Verification items for the finished model (mm, model axes). A direction names the side the tool comes from. Coordinates: 2 decimals unless noted, no trailing zeros. Order: outer loops, then holes, each group sorted by start corner. A loop starts at its lowest first (then second) coordinate and runs counter-clockwise, first axis right, second up. Notation, with made-up numbers: M -14,4 L -5,4 A18 ccw -5,21 Z; hole C 71.5,5 d11. An arc over 180 degrees is marked long. Return JSON: item names as keys, results as strings. Group by question number.
1. Section check D-D, the plane y = 3.9. Record the cut outline in (x, z), plus the area to 3 significant figures.
2. Section check A-A, the plane z = 2. Record the cut outline in (x, y), plus the area to 3 significant figures.
3. Section check C-C, the plane y = 2.1. Record the cut outline in (x, z).
4. Material ranges on line 1 along Y through (x, z) = (-1.25, 4.75); line 2 along X through (y, z) = (1.2, 9); line 3 along X through (y, z) = (1.7, 1), recorded low to high.
5. Set-up check for faces 4 (the flat face through (0, 3, 0)), 5 (the cylindrical face through (0, 2.8, 4.9)): record each of +Z, -Z, +X, -X, +Y, -Y from which the full face is reachable in a straight line by a thin tool's end or side.
6. Mould release check, pull along X, two halves, no side actions. Record for faces 1 (the flat face through (0.708, 2.008, 4.93)), 2 (the cylindrical face through (-4.715, 0.301, 5.07)), 3 (the cylindrical face through (4.699, 0.285, 5.07)): +X half, -X half, draft (parallel to the pull), parting line (faces both ways), or undercut.
7. Section check B-B, the plane x = 0. Record the cut outline in (y, z), plus the area to 3 significant figures.
Autodesk Inventor part; units mm, degrees
ref_plane "YZ Plane" through (0, 0, 0) normal (1, 0, 0) x (0, 1, 0)
ref_plane "XZ Plane" through (0, 0, 0) normal (0, 1, 0) x (-1, 0, 0)
ref_plane "XY Plane" through (0, 0, 0) normal (0, 0, 1) x (1, 0, 0)
sketch "Sketch1" plane through (0, 0, 0) normal (0, 0, 1) x (1, 0, 0)
  line L0 (-5, 0) -> (5, 0)
  line L1 (5, 0) -> (5, 4.3)
  line L2 (5, 4.3) -> (-5, 4.3)
  line L3 (-5, 4.3) -> (-5, 0)
  line L4 (-3.75, 0) -> (3.75, 0)
  line L5 (3.75, 0) -> (3.75, 1.6)
  line L6 (3.75, 1.6) -> (-3.75, 1.6)
  line L7 (-3.75, 1.6) -> (-3.75, 0)
  line L8 (-3.75, 1) -> (3.75, 1)
  circle A0 centre (0, 2.2) radius 0.6
  line L9 (-0.5638, 2.4052) -> (-0.8569, 1.6)
  line L10 (0.5638, 2.4052) -> (0.8569, 1.6)
  point P0 (0, 0)
  dimension "d0" = 10
  dimension "d1" = 7.5
  dimension "d2" = 3.75
  dimension "d3" = 5
  dimension "d4" = 1
  dimension "d5" = 0.6
  dimension "d6" = 1.2
  dimension "d7" = 1.5
  dimension "d8" = 70
  dimension "d9" = 70
extrude "Extrusion1" add sketch "Sketch1" along normal blind 10 contours L3 L2 L1 L0 L5 L6 L10 A0 L9 L7 | L7 L8 L5 L0
fillet "Fillet1" radius 1 4 edges at (5, 4.3, 5) (5, 0, 5) (-5, 4.3, 5) (-5, 0, 5)
properties part number "Cable_tie_attachment"
Answers follow:
{
 "1": {"outline": "M -4.8,0 L 4.8,0 L 4.8,10 L -4.8,10 Z", "area": "96.0 mm^2"},
 "2": {"outline": "M -5,1 A1 ccw -4,0 L 4,0 A1 ccw 5,1 L 5,3.3 A1 ccw 4,4.3 L -4,4.3 A1 ccw -5,3.3 Z; hole M -3.75,1 L 3.75,1 L 3.75,1.6 L 0.86,1.6 L 0.56,2.41 A0.6 ccw -0.56,2.41 L -0.86,1.6 L -3.75,1.6 Z", "area": "36.2 mm^2"},
 "3": {"outline": "M -5,0 L -0.67,0 L -0.67,10 L -5,10 Z; M 0.67,0 L 5,0 L 5,10 L 0.67,10 Z"},
 "4": {"line 1": "0 to 1, 1.6 to 4.3", "line 2": "-5 to -3.75, 3.75 to 5", "line 3": "-5 to -0.82, 0.82 to 5"},
 "5": {"face 4": "-Z, +X, -X, +Y, -Y", "face 5": "+Z, -Z"},
 "6": {"face 1": "undercut", "face 2": "-X half", "face 3": "+X half"},
 "7": {"outline": "M 0,0 L 1,0 L 1,10 L 0,10 Z; M 2.8,0 L 4.3,0 L 4.3,10 L 2.8,10 Z", "area": "25.0 mm^2"}
}
